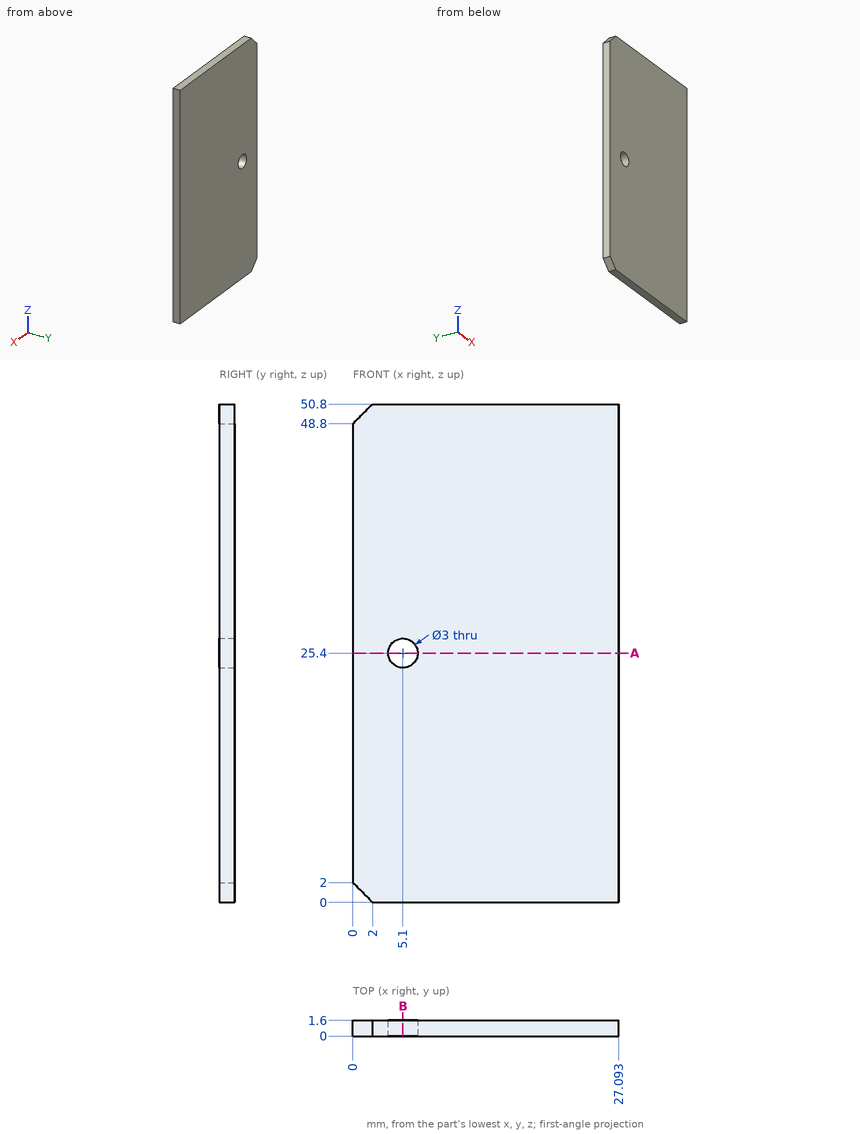
Could you check a few things on this drawing? It's one solid part, dimensions in mm from its lowest x, y, z. Give positions to 0.01 mm unless a question says otherwise; leave off trailing zeros. Order: outer loops, then holes, each group sorted by start corner. A loop starts at its lowest first (then second) coordinate and runs counter-clockwise, first axis right, second up. Notation, with made-up numbers: (29, 8) - (78, 8) arc R12 ccw to (78, 23) - close; hole circle Ø11 at (52, 17.25). An arc over 180 degrees is marked (long way). One line per question, with ' | ' between items. Start each with the question number.
Item 1: I need wall thicknesses on probe 1 along X at (y, z) = (1.05, 25.4); probe 2 along Z at (x, y) = (1, 0.75). Which ranges of each line are inside material? Lowest first, please. Write a range as [from, to].
Item 2: I'm going to push a flat-ended pin straight in: pin 1 Ø1.8 at (x, z) = (5.1, 25.4) entering from -Y. Where does the tip first touch, or does it pass through?
Item 3: I want a section at A-A on z = 25.4. Write out the boundary of the cut face in (x, y).
Item 4: I want a section at B-B on x = 5.1. Write out the boundary of the cut face in (y, z).
Verdict:
1) probe 1: [0, 3.6], [6.6, 27.09] | probe 2: [1, 49.8]
2) pin 1: through
3) outline: (0, 0) - (3.6, 0) - (3.6, 1.6) - (0, 1.6) - close; (6.6, 0) - (27.09, 0) - (27.09, 1.6) - (6.6, 1.6) - close
4) outline: (0, 0) - (1.6, 0) - (1.6, 23.9) - (0, 23.9) - close; (0, 26.9) - (1.6, 26.9) - (1.6, 50.8) - (0, 50.8) - close
